Autodesk Inventor part; units mm, degrees
ref_plane "YZ Plane" through (0, 0, 0) normal (1, 0, 0) x (0, 1, 0)
ref_plane "XZ Plane" through (0, 0, 0) normal (0, 1, 0) x (-1, 0, 0)
ref_plane "XY Plane" through (0, 0, 0) normal (0, 0, 1) x (1, 0, 0)
sketch "Boceto1" plane through (0, 0, 0) normal (1, 0, 0) x (0, 1, 0)
  line L0 (0, 0) -> (40, 0)
  line L1 (40, 0) -> (40, -90)
  line L2 (40, -90) -> (0, -90)
  line L3 (0, -90) -> (0, 0)
  dimension "d0" = 40
  dimension "d1" = 90
extrude "Extrusión1" add sketch "Boceto1" along normal blind 5
sketch "Boceto2" plane through (0, 0, 0) normal (0, 0, 1) x (1, 0, 0)
  circle A0 centre (2.5, 5) radius 1.5
  circle A1 centre (2.5, 35) radius 1.5
  line L0 (0, 40) -> (0, 0)
  line L1 (0, 40) -> (5, 40)
  line L2 (0, 0) -> (5, 0)
  line L3 (5, 40) -> (5, 0)
  point P0 (2.5, 0)
  dimension "d4" = 3
  dimension "d5" = 3
  dimension "d6" = 2.5
  dimension "d7" = 5
  dimension "d8" = 5
  dimension "d9" = 2.5
extrude "Extrusión2" cut sketch "Boceto2" against normal blind 3 contours A0 | A1
sketch "Boceto3" plane through (0, 0, -90) normal (0, 0, -1) x (-1, 0, 0)
  circle A0 centre (-2.5, 5) radius 1.5
  circle A1 centre (-2.5, 5) radius 1.5
  circle A2 centre (-2.5, 35) radius 1.5
  circle A3 centre (-2.5, 35) radius 1.5
  point P0 (0, 0)
extrude "Extrusión3" cut sketch "Boceto3" against normal blind 3
properties part number "Frontal"
For this review, take the finished solid that the model builds, in its own axes (mm). A direction names the side the tool comes from. Round coordinates to 2 decimals unless told otherwise and drop trailing zeros. Order: outer loops, then holes, each group sorted by start corner. A loop starts at its lowest first (then second) coordinate and runs counter-clockwise, first axis right, second up. Notation, with made-up numbers: (0, 12.5) -> (13, 12.5) arc R22 cw to (13, 41.5) -> close; hole circle Ø11 at (77, 86). An arc over 180 degrees is marked (long way). Use a Markdown table: item, result.
Item 1: Machinability: for faces 1 (the flat face through (3, 35, -87)), 2 (the cylindrical face through (2.175, 33.536, -1.479)), 3 (the flat face through (2, 40, -44)), which of the approach directions +Z, -Z, +X, -X, +Y, -Y give a long, thin tool a straight path to every point of the face, cutting with its end or side? Answer none if there is none.
Resolved:
| item | result |
|---|---|
| face 1 | -Z |
| face 2 | +Z |
| face 3 | +Z, -Z, +X, -X, +Y |
Item 2: For line 1 along Y through (x, z) = (2.5, -89.3); line 2 along Z through (x, y) = (2.35, 5.5), list the stretches that pass through material, from the lowest coordinate up. Write a range as [from, to].
Resolved:
| item | result |
|---|---|
| line 1 | y = [0, 3.5], [6.5, 33.5], [36.5, 40] |
| line 2 | z = [-87, -3] |
Item 3: For pin 1 (0.9 mm diameter, centred on x = 2, y = 4.5, fed in from -Z); pin 2 (1.8 mm diameter, centred on x = 2.5, y = 35, fed in from +Z), all flat-tipped, find the tip position at first contact; note any pin that passes through.
Resolved:
| item | result |
|---|---|
| pin 1 | stops at z = -87 |
| pin 2 | stops at z = -3 |
Item 4: Draft analysis for pull direction X (two halves, no side actions). For faces 4 (the cylindrical face through (1, 5, -89)), 5 (the flat face through (0, 20, -44)), 6 (the flat face through (2, 0, -46)), state which applies: +X half, -X half, draft (parallel to the pull), parting line (faces both ways), or undercut.
Resolved:
| item | result |
|---|---|
| face 4 | undercut |
| face 5 | -X half |
| face 6 | draft |
Item 5: Take a section at A-A (y = 5). State the section outline as (x, z) points.
Resolved:
| item | result |
|---|---|
| outline | (0, -90) -> (1, -90) -> (1, -87) -> (4, -87) -> (4, -90) -> (5, -90) -> (5, 0) -> (4, 0) -> (4, -3) -> (1, -3) -> (1, 0) -> (0, 0) -> close |
